Design review of the part built by this model. Coordinates are the model's own, in mm. Coordinates: 2 decimals unless noted, no trailing zeros. Loops run counter-clockwise (first coordinate to the right, second up) from the corner with the lowest first, then second, coordinate; pieces in that order, holes last. Notation, with made-up numbers: (-13.5, 28.5) - (27.5, 28.5) arc R23 cw to (27.5, 63.5) - close; hole circle Ø2 at (1, 3). An arc over 180 degrees is marked (long way). Use one line per item in the form item = value. Start each with the question number.
(1) Clearance check with a flat-ended pin moving along its axis: pin 1 Ø1.2 at (x, z) = (-7.96, 18.99) entering from -Y. State where the tip first meets the part, or that it passes through.
(2) Add section A-A (z = 0). State the section outline as (x, y) points, plus the area to 3 significant figures.
(3) For L1, parallel to X at y = 3.4, z = 19; L2, parallel to X at y = 0.1, z = 0; L3, parallel to Y at x = -4, z = 4.75, list the stretches that pass through material, from the lowest coordinate up.
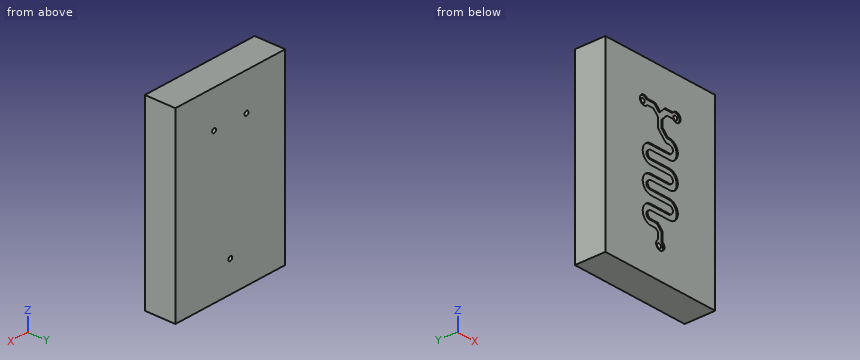
Autodesk Inventor part; units mm, degrees
ref_plane "YZ Plane" through (0, 0, 0) normal (1, 0, 0) x (0, 1, 0)
ref_plane "XZ Plane" through (0, 0, 0) normal (0, 1, 0) x (-1, 0, 0)
ref_plane "XY Plane" through (0, 0, 0) normal (0, 0, 1) x (1, 0, 0)
sketch "Boceto1" plane through (0, 0, 0) normal (0, 1, 0) x (-1, 0, 0)
  line L0 (3.5954, 15.5561) -> (3.1417, 15.5533)
  line L1 (3.3005, 14.6566) -> (3.9682, 14.6566)
  line L2 (5.45, 1.7061) -> (5.45, 0.6)
  line L3 (3.5954, 15.5561) -> (4.55, 16.5107)
  line L4 (4.55, 16.5107) -> (4.55, 17.7346)
  line L5 (5.45, 17.735) -> (5.45, 16.1384)
  line L6 (5.45, 16.1384) -> (3.9682, 14.6566)
  line L7 (6.6995, 10.4566) -> (3.3005, 10.4566)
  line L8 (3.3005, 11.3566) -> (6.6995, 11.3566)
  arc A0 (6.6995, 11.3566) -> (6.6995, 12.5566) centre (6.6995, 11.9566) ccw
  arc A1 (6.6995, 10.4566) -> (6.6995, 13.4566) centre (6.6995, 11.9566) ccw
  line L9 (6.6995, 12.5566) -> (3.3005, 12.5566)
  arc A2 (3.3005, 14.6566) -> (3.3005, 13.4566) centre (3.3005, 14.0566) ccw
  arc A3 (3.1417, 15.5533) -> (3.3005, 12.5566) centre (3.3026, 14.0593) ccw
  line L10 (3.3005, 13.4566) -> (6.6995, 13.4566)
  line L11 (3.3005, 9.2566) -> (6.6995, 9.2566)
  arc A4 (3.3005, 10.4566) -> (3.3005, 9.2566) centre (3.3005, 9.8566) ccw
  arc A5 (3.3005, 11.3566) -> (3.3005, 8.3566) centre (3.3005, 9.8566) ccw
  line L12 (6.6995, 8.3566) -> (3.3005, 8.3566)
  arc A6 (6.6995, 7.1566) -> (6.6995, 8.3566) centre (6.6995, 7.7566) ccw
  arc A7 (6.6995, 6.2566) -> (6.6995, 9.2566) centre (6.6995, 7.7566) ccw
  line L13 (3.3005, 7.1566) -> (6.6995, 7.1566)
  line L14 (6.6995, 6.2566) -> (3.3005, 6.2566)
  arc A8 (3.3005, 6.2566) -> (3.3005, 5.0566) centre (3.3005, 5.6566) ccw
  arc A9 (3.3005, 7.1566) -> (3.3005, 4.1566) centre (3.3005, 5.6566) ccw
  line L15 (3.3005, 5.0566) -> (6.6995, 5.0566)
  line L16 (6.6995, 4.1566) -> (3.3005, 4.1566)
  arc A10 (6.6995, 2.9566) -> (6.6995, 4.1566) centre (6.6995, 3.5566) ccw
  arc A11 (6.6995, 2.0566) -> (6.6995, 5.0566) centre (6.6995, 3.5566) ccw
  line L17 (4.55, 2.0789) -> (5.4276, 2.9566)
  line L18 (6.6995, 2.0566) -> (5.8004, 2.0566)
  line L19 (5.8004, 2.0566) -> (5.45, 1.7061)
  line L20 (4.55, 0.6) -> (4.55, 2.0789)
  arc A12 (4.55, 0.6) -> (5.45, 0.6) centre (5, 0) ccw
  line L21 (5.4276, 2.9566) -> (6.6995, 2.9566)
  line L22 (15, -5) -> (15, 25)
  line L23 (15, 25) -> (-5, 25)
  line L24 (-5, 25) -> (-5, -5)
  line L25 (-5, -5) -> (15, -5)
  line L26 (3.7496, 18.535) -> (2.6434, 18.535)
  line L27 (4.1224, 19.435) -> (4.9998, 18.5576)
  line L28 (4.55, 17.7346) -> (3.7496, 18.535)
  line L29 (2.6434, 19.435) -> (4.1224, 19.435)
  arc A13 (2.6434, 19.435) -> (2.6434, 18.535) centre (2.0434, 18.985) ccw
  line L30 (6.2504, 18.5355) -> (7.3566, 18.5355)
  line L31 (7.3566, 19.4355) -> (5.8776, 19.4355)
  arc A14 (7.3566, 18.5355) -> (7.3566, 19.4355) centre (7.9566, 18.9855) ccw
  line L32 (5.45, 17.735) -> (6.2504, 18.5355)
  line L33 (5.8776, 19.4355) -> (4.9998, 18.5576)
extrude "Extrusión1" add sketch "Boceto1" along normal blind 5 contours L3 L4 L28 L26 A13 L29 L27 L33 L31 A14 L30 L32 L5 L6 L1 A2 L10 A1 L7 A4 L11 A7 L14 A8 L15 A11 L18 L19 L2 A12 L20 L17 L21 A10 L16 A9 L13 A6 L12 A5 L8 A0 L9 A3 L0 | L25 L24 L23 L22
extrude "Extrusión2" cut sketch "Boceto1" along normal blind 0.2 contours L3 L4 L28 L26 A13 L29 L27 L33 L31 A14 L30 L32 L5 L6 L1 A2 L10 A1 L7 A4 L11 A7 L14 A8 L15 A11 L18 L19 L2 A12 L20 L17 L21 A10 L16 A9 L13 A6 L12 A5 L8 A0 L9 A3 L0
sketch "Boceto3" plane through (0, 0.2, 0) normal (0, -1, 0) x (1, 0, 0)
  arc A0 (-2.6434, 18.535) -> (-2.6434, 19.435) centre (-2.0434, 18.985) ccw
  arc A1 (-7.3566, 19.4355) -> (-7.3566, 18.5355) centre (-7.9566, 18.9855) ccw
  arc A2 (-5.45, 0.6) -> (-4.55, 0.6) centre (-5, 0) ccw
  circle A3 centre (-2.0434, 18.985) radius 0.35
  circle A4 centre (-7.9566, 18.985) radius 0.35
  circle A5 centre (-5, 0) radius 0.35
  point P0 (0, 0)
  dimension "d5" = 0.7
  dimension "d6" = 0.7
  dimension "d7" = 0.7
extrude "Extrusión3" cut sketch "Boceto3" against normal through all
properties part number "Mixer"
Computed values:
q1.pin_1 = 0.2
q2.outline = (-15, 0) - (-5.75, 0) - (-5.75, 0.2) - (-5.35, 0.2) - (-5.35, 5) - (-15, 5) - close; (-4.65, 0.2) - (-4.25, 0.2) - (-4.25, 0) - (5, 0) - (5, 5) - (-4.65, 5) - close
q2.area = 96.3 mm^2
q3.L1 = -15 to -8.31, -7.61 to -2.39, -1.69 to 5
q3.L2 = -15 to -5.75, -4.25 to 5
q3.L3 = 0.2 to 5
